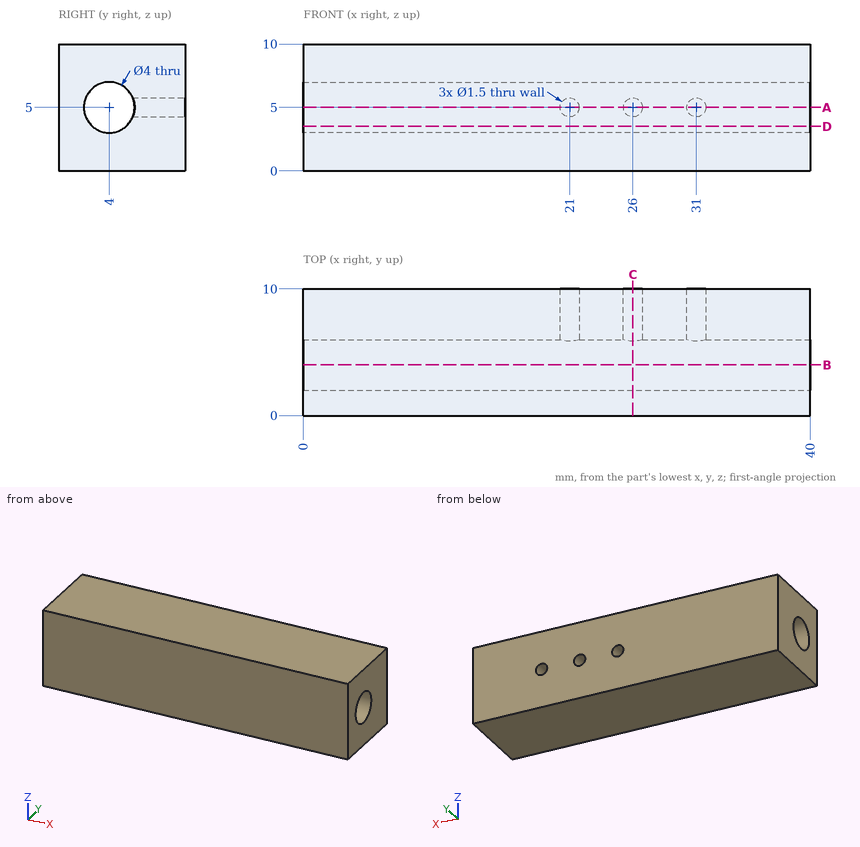
Geometry: see drawing. Coordinates: mm, zero at the bounding-box minimum. Give positions to 0.01 mm unless a question says otherwise; leave off trailing zeros. Write each loop counter-clockwise with the first axis right and the second up, starting at its lowest first coordinate (ties: lowest second). Pieces come first, ordered by that corner, then holes. Notation, with made-up numbers: M 7,14.5 L 20,14.5 A36 ccw 20,48.5 Z; hole C -25.75,-23 d6. An arc over 180 degrees is marked long. Answer in a Markdown table with one row per item. Add a question column.
(1) Section D-D on z = 3.5. Return loops of the section in (x, y).
(2) First-contact query: pin 1 (2 mm diameter, centred on x = 35.5, y = 1, fed in from -Z); pin 2 (0.9 mm diameter, centred on x = 31, z = 5, fed in from +Y). Flat tips, straight axial feed; report the tip coordinate or a pass-through.
(3) Section C-C on x = 26. Return loops of the section in (y, z), and give its area (3 significant figures).
(4) Section A-A on z = 5. Return loops of the section in (x, y), and give its area (3 significant figures).
(5) Ray query, line 1 (X direction, y = 7.85, z = 5); line 2 (Z direction, x = 31, y = 9); line 3 (Y direction, x = 6.5, z = 4.75). Return the intervals inside material, ascending.
(6) Section B-B on y = 4. Return loops of the section in (x, z), and give its area (3 significant figures).
Result set:
| question | item | result |
|---|---|---|
| 1 | outline | M 0,0 L 40,0 L 40,2.68 L 0,2.68 Z; M 0,5.32 L 40,5.32 L 40,10 L 0,10 Z |
| 2 | pin 1 | stops at z = 0 |
| 2 | pin 2 | stops at y = 2.05 |
| 3 | outline | M 0,0 L 10,0 L 10,4.25 L 5.85,4.25 A2 cw long 5.85,5.75 L 10,5.75 L 10,10 L 0,10 Z |
| 3 | area | 81.4 mm^2 |
| 4 | outline | M 0,0 L 40,0 L 40,2 L 0,2 Z; M 0,6 L 20.25,6 L 20.25,10 L 0,10 Z; M 21.75,6 L 25.25,6 L 25.25,10 L 21.75,10 Z; M 26.75,6 L 30.25,6 L 30.25,10 L 26.75,10 Z; M 31.75,6 L 40,6 L 40,10 L 31.75,10 Z |
| 4 | area | 222 mm^2 |
| 5 | line 1 | x = 0 to 20.25, 21.75 to 25.25, 26.75 to 30.25, 31.75 to 40 |
| 5 | line 2 | z = 0 to 4.25, 5.75 to 10 |
| 5 | line 3 | y = 0 to 2.02, 5.98 to 10 |
| 6 | outline | M 0,0 L 40,0 L 40,3 L 0,3 Z; M 0,7 L 40,7 L 40,10 L 0,10 Z |
| 6 | area | 240 mm^2 |
